Part model, mm, in its own coordinate system. Face numbers are marked on the shaded views. A direction names the side the tool comes from. Coordinates: 2 decimals unless noted, no trailing zeros. Loops run counter-clockwise (first coordinate to the right, second up) from the corner with the lowest first, then second, coordinate; pieces in that order, holes last. Notation, with made-up numbers: M -13,-22 L 34,-22 A18 ccw 34,-2 Z; hole C 1,40.5 d3. An arc over 180 degrees is marked long. Answer as a JSON object with one key per item and string values. Group by question number.
1. Drill centre lines: L1, parallel to X at y = 29.5, z = 11.75; L2, parallel to X at y = -51, z = 11.75; L3, parallel to Y at x = -40.5, z = 8 (3 decimals). Where is each one in solid material? Low to high.
2. Saw through at C-C on z = 2.75. Write the cut outline in (x, y), then the cut area to 3 significant figures.
3. Drop flat-ended pins along their axis: pin 1 Ø19 at (x, y) = (-23.5, 28) entering from +Z; pin 2 Ø4 at (x, z) = (18, 10) entering from -Y; pin 3 Ø3 at (x, z) = (23, 5.5) entering from -Y. Give the stop position or say it passes through.
4. Saw through at D-D on x = 15.5. Write the cut outline in (y, z) (3 decimals), then the cut area to 3 significant figures.
5. Mould opens along X. For the marked faces 3, 4 and 5 say: released by +X, released by -X, zero draft, split by the parting line, or undercut.
6. 3-axis set-ups, long thin cutter, end or side, ignore diameter. For the marked faces 1 and 2: which of +Z, -Z, +X, -X, +Y, -Y reach the whole face in a straight line?
7. Saw through at B-B on z = 9. Write the cut outline in (x, y), then the cut area to 3 significant figures.
8. Saw through at A-A on y = 11. Write the cut outline in (x, z).
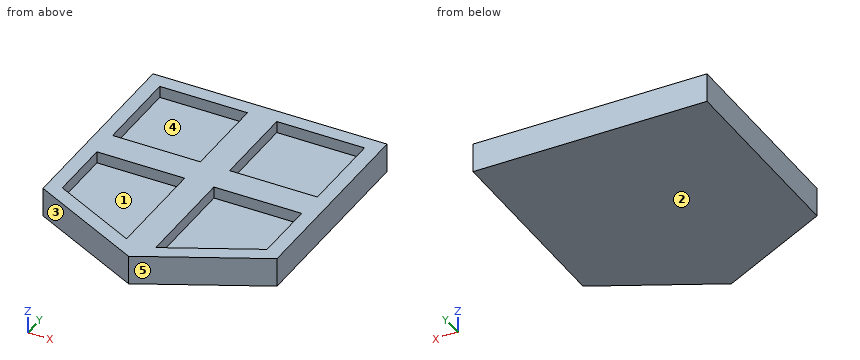
from build123d import *

# Parameters (mm, degrees)
F0_W     = 50.8
F0_H     = 50.8
F1_DEPTH = 12.7
F2_W     = 38.1
F2_H     = 38.1
F4_DEPTH = 5.08
F5_DEPTH = 5.08


with BuildPart() as f1:
    # F0 (on Top) → F1 (new body)
    with BuildSketch(Plane.XY):
        with Locations((-25.4, 25.4)):
            Rectangle(F0_W, F0_H)
        with Locations((25.4, 25.4)):
            Rectangle(F0_W, F0_H)
        Polygon((50.8, 0), (0, 0), (0, -63.5), (50.8, -38.1), align=None)
        Polygon((0, -63.5), (0, 0), (-50.8, 0), (-50.8, -38.1), align=None)
    extrude(amount=F1_DEPTH)

    # F2 (on face) → F4 (cut)
    with BuildSketch(Plane.XY.offset(12.7)):
        with Locations((-25.4, 25.4)):
            Rectangle(F2_W, F2_H)
        with Locations((25.4, 25.4)):
            Rectangle(F2_W, F2_H)
    extrude(amount=-F4_DEPTH, mode=Mode.SUBTRACT)

    # F3 (on face) → F5 (cut)
    with BuildSketch(Plane.XY.offset(12.7)):
        Polygon((-6.35, -6.35), (-44.45, -6.35), (-44.45, -34.29), (-6.35, -53.34), align=None)
        Polygon((6.35, -6.35), (6.35, -53.34), (44.45, -34.29), (44.45, -6.35), align=None)
    extrude(amount=-F5_DEPTH, mode=Mode.SUBTRACT)


solid = f1.part
Outcome:
{
 "1": {"L1": "x = -50.8 to -44.45, -6.35 to 6.35, 44.45 to 50.8", "L2": "x = -25 to -11.03, -6.35 to 6.35, 11.03 to 25", "L3": "y = -43.25 to -36.265, -6.35 to 6.35, 44.45 to 50.8"},
 "2": {"outline": "M -50.8,-38.1 L 0,-63.5 L 50.8,-38.1 L 50.8,50.8 L -50.8,50.8 Z", "area": "10,300 mm²"},
 "3": {"pin 1": "stops at z = 7.62", "pin 2": "stops at y = -55.5", "pin 3": "stops at y = -52.75"},
 "4": {"outline": "M -55.75,0 L 50.8,0 L 50.8,12.7 L 44.45,12.7 L 44.45,7.62 L 6.35,7.62 L 6.35,12.7 L -6.35,12.7 L -6.35,7.62 L -48.765,7.62 L -48.765,12.7 L -55.75,12.7 Z", "area": "944 mm²"},
 "5": {"face 3": "released by -X", "face 4": "undercut", "face 5": "released by +X"},
 "6": {"face 1": "+Z", "face 2": "-Z, +X, -X, +Y, -Y"},
 "7": {"outline": "M -50.8,-38.1 L 0,-63.5 L 50.8,-38.1 L 50.8,50.8 L -50.8,50.8 Z; hole M -44.45,-34.29 L -6.35,-53.34 L -6.35,-6.35 L -44.45,-6.35 Z; hole M -44.45,6.35 L -6.35,6.35 L -6.35,44.45 L -44.45,44.45 Z; hole M 6.35,-53.34 L 44.45,-34.29 L 44.45,-6.35 L 6.35,-6.35 Z; hole M 6.35,6.35 L 44.45,6.35 L 44.45,44.45 L 6.35,44.45 Z", "area": "4,560 mm²"},
 "8": {"outline": "M -50.8,0 L 50.8,0 L 50.8,12.7 L 44.45,12.7 L 44.45,7.62 L 6.35,7.62 L 6.35,12.7 L -6.35,12.7 L -6.35,7.62 L -44.45,7.62 L -44.45,12.7 L -50.8,12.7 Z"}
}
